from build123d import *

# Parameters (mm, degrees)
ESQUISSE1_W                  = 50
ESQUISSE1_H                  = 100
BOSS_EXTRU_1_DEPTH           = 51.25
ESQUISSE2_W                  = 40
ESQUISSE2_H                  = 40
ESQUISSE2_W_2                = 20
ESQUISSE2_H_2                = 20
BOSS_EXTRU_2_DEPTH           = 45.5
BOSS_EXTRU_2_DEPTH_BACK      = 100
ESQUISSE2_3_W                = 40
ESQUISSE2_3_H                = 82.5
ENL_V_MAT_EXTRU_1_DEPTH      = 101
ENL_V_START                  = -2.5
ENL_V_MAT_EXTRU_3_DEPTH      = 49.75
ENL_V_START_2                = 2.5
ENL_V_MAT_EXTRU_4_DEPTH      = 49.75
ESQUISSE1_6_R                = 5
ENL_V_MAT_EXTRU_5_DEPTH      = 52.25
ENL_V_MAT_EXTRU_5_DEPTH_BACK = 52.25
ENL_V_START_3                = -20
ESQUISSE1_7_W                = 20
ESQUISSE1_7_H                = 85.5
ENL_V_MAT_EXTRU_6_DEPTH      = 31.25
ENL_V_START_4                = 20
ESQUISSE1_8_W                = 20
ESQUISSE1_8_H                = 85.5
ENL_V_MAT_EXTRU_7_DEPTH      = 31.25


with BuildPart() as part:
    # Esquisse1 → Boss.-Extru.1 (new body, symmetric)
    with BuildSketch(Plane.XY):
        with Locations((-25, 50)):
            Rectangle(ESQUISSE1_W, ESQUISSE1_H)
    extrude(amount=BOSS_EXTRU_1_DEPTH, both=True)

    # Esquisse2 → Boss.-Extru.2 (add, two sides)
    with BuildSketch(Plane(origin=(0, 100, 0), x_dir=(1, 0, 0), z_dir=(0, 1, 0))) as boss_extru_2_sk:
        Polygon((205, 20), (50, 44.340452261), (50, -44.340452261), (205, -20), (185, -20), (185, 20), align=None)
        Polygon((6, 51.25), (0, 51.25), (0, 41.25), (40, 41.25), (40, -41.25), (0, -41.25), (0, -51.25), (6, -51.25), (50, -44.340452261), (50, 44.340452261), align=None)
        with Locations((205, 0)):
            Rectangle(ESQUISSE2_W, ESQUISSE2_H)
        with Locations((205, 0)):
            Rectangle(ESQUISSE2_W_2, ESQUISSE2_H_2, mode=Mode.SUBTRACT)
    extrude(amount=BOSS_EXTRU_2_DEPTH)
    extrude(boss_extru_2_sk.sketch, amount=-BOSS_EXTRU_2_DEPTH_BACK)

    # Esquisse2_3 → Enl_v. mat.-Extru.1 (cut, through all)
    with BuildSketch(Plane(origin=(0, 100, 0), x_dir=(1, 0, 0), z_dir=(0, 1, 0))):
        with Locations((-20, 0)):
            Rectangle(ESQUISSE2_3_W, ESQUISSE2_3_H)
        with Locations((20, 0)):
            Rectangle(ESQUISSE2_3_W, ESQUISSE2_3_H)
    extrude(amount=-ENL_V_MAT_EXTRU_1_DEPTH, mode=Mode.SUBTRACT)

    # Esquisse1_4 → Enl_v. mat.-Extru.3 (cut, through all)
    with BuildSketch(Plane.XY.offset(ENL_V_START)):
        with BuildLine():
            Line((50, 100), (50, 20))
            Line((50, 20), (65, 20))
            ThreePointArc((65, 20), (72.071067812, 17.071067812), (75, 10))
            Line((75, 10), (75, 6))
            Line((75, 6), (103.975092222, 6))
            ThreePointArc((103.975092222, 6), (108.20127484, 6.93692213), (111.635536654, 9.572123903))
            Line((111.635536654, 9.572123903), (139.204786201, 42.427876097))
            ThreePointArc((139.204786201, 42.427876097), (142.639048015, 45.06307787), (146.865230633, 46))
            Line((146.865230633, 46), (165, 46))
            Line((165, 46), (165, 50))
            ThreePointArc((165, 50), (167.928932188, 57.071067812), (175, 60))
            Line((175, 60), (185, 60))
            Line((185, 60), (185, 145.5))
            Line((185, 145.5), (171.285964092, 145.5))
            ThreePointArc((171.285964092, 145.5), (167.059781475, 144.56307787), (163.625519661, 141.927876097))
            Line((163.625519661, 141.927876097), (131.441222142, 103.572123903))
            ThreePointArc((131.441222142, 103.572123903), (128.006960328, 100.93692213), (123.780777711, 100))
            Line((123.780777711, 100), (50, 100))
        make_face()
    extrude(amount=-ENL_V_MAT_EXTRU_3_DEPTH, mode=Mode.SUBTRACT)

    # Esquisse1_5 → Enl_v. mat.-Extru.4 (cut, through all)
    with BuildSketch(Plane.XY.offset(ENL_V_START_2)):
        with BuildLine():
            Line((50, 100), (50, 20))
            Line((50, 20), (65, 20))
            ThreePointArc((65, 20), (72.071067812, 17.071067812), (75, 10))
            Line((75, 10), (75, 6))
            Line((75, 6), (103.975092222, 6))
            ThreePointArc((103.975092222, 6), (108.20127484, 6.93692213), (111.635536654, 9.572123903))
            Line((111.635536654, 9.572123903), (139.204786201, 42.427876097))
            ThreePointArc((139.204786201, 42.427876097), (142.639048015, 45.06307787), (146.865230633, 46))
            Line((146.865230633, 46), (165, 46))
            Line((165, 46), (165, 50))
            ThreePointArc((165, 50), (167.928932188, 57.071067812), (175, 60))
            Line((175, 60), (185, 60))
            Line((185, 60), (185, 145.5))
            Line((185, 145.5), (171.285964092, 145.5))
            ThreePointArc((171.285964092, 145.5), (167.059781475, 144.56307787), (163.625519661, 141.927876097))
            Line((163.625519661, 141.927876097), (131.441222142, 103.572123903))
            ThreePointArc((131.441222142, 103.572123903), (128.006960328, 100.93692213), (123.780777711, 100))
            Line((123.780777711, 100), (50, 100))
        make_face()
    extrude(amount=ENL_V_MAT_EXTRU_4_DEPTH, mode=Mode.SUBTRACT)

    # Esquisse1_6 → Enl_v. mat.-Extru.5 (cut, two sides)
    with BuildSketch(Plane.XY) as enl_v_mat_extru_5_sk:
        with BuildLine():
            Line((0, 100), (50, 100))
            Line((50, 100), (123.780777711, 100))
            ThreePointArc((123.780777711, 100), (128.006960328, 100.93692213), (131.441222142, 103.572123903))
            Line((131.441222142, 103.572123903), (163.625519661, 141.927876097))
            ThreePointArc((163.625519661, 141.927876097), (167.059781475, 144.56307787), (171.285964092, 145.5))
            Line((171.285964092, 145.5), (0, 145.5))
            Line((0, 145.5), (0, 100))
        make_face()
        with BuildLine():
            ThreePointArc((114.433382603, 3.572123903), (110.999120789, 0.93692213), (106.772938171, 0))
            Line((106.772938171, 0), (225, 0))
            Line((225, 0), (225, 40))
            Line((225, 40), (205, 40))
            Line((205, 40), (149.663076582, 40))
            ThreePointArc((149.663076582, 40), (145.436893964, 39.06307787), (142.00263215, 36.427876097))
            Line((142.00263215, 36.427876097), (114.433382603, 3.572123903))
        make_face()
        with Locations((65, 10)):
            Circle(ESQUISSE1_6_R)
        with Locations((175, 50)):
            Circle(ESQUISSE1_6_R)
    extrude(amount=ENL_V_MAT_EXTRU_5_DEPTH, mode=Mode.SUBTRACT)
    extrude(enl_v_mat_extru_5_sk.sketch, amount=-ENL_V_MAT_EXTRU_5_DEPTH_BACK, mode=Mode.SUBTRACT)

    # Esquisse1_7 → Enl_v. mat.-Extru.6 (cut)
    with BuildSketch(Plane.XY.offset(ENL_V_START_3)):
        with Locations((195, 102.75)):
            Rectangle(ESQUISSE1_7_W, ESQUISSE1_7_H)
    extrude(amount=-ENL_V_MAT_EXTRU_6_DEPTH, mode=Mode.SUBTRACT)

    # Esquisse1_8 → Enl_v. mat.-Extru.7 (cut)
    with BuildSketch(Plane.XY.offset(ENL_V_START_4)):
        with Locations((195, 102.75)):
            Rectangle(ESQUISSE1_8_W, ESQUISSE1_8_H)
    extrude(amount=ENL_V_MAT_EXTRU_7_DEPTH, mode=Mode.SUBTRACT)


solid = part.part
Can you work these out from the model? Positions are in its coordinate system, mm. A direction names the side the tool comes from. Coordinates: 2 decimals unless noted, no trailing zeros. Order: outer loops, then holes, each group sorted by start corner. A loop starts at its lowest first (then second) coordinate and runs counter-clockwise, first axis right, second up. Notation, with made-up numbers: (18, -24.75) - (66, -24.75) arc R18 cw to (66, -16.75) - close; hole circle Ø6 at (26, 29). An arc over 180 degrees is marked (long way). Answer as a JSON object with one key per item and string values. Group by question number.
Q1. Imagine slicing it at C-C (y = 110.5). Please give me the cut outline in (x, z), and give its area (3 significant figures).
Q2. We'd pull the mould along Z, two halves only. Please class faces 1 (the face through (215, 93, 0)), 2 (the face through (89, 6, -21)): +Z half, -Z half, draft (parallel to the pull), parting line (faces both ways), or undercut.
Q3. I need wall thicknesses on line 1 (X direction, y = 96, z = -17.5); line 2 (X direction, y = 96.5, z = -2); line 3 (X direction, y = 50, z = 3). Which ranges of each line are inside material? Lowest first, please. Write a range as from..to.
Q4. Imagine slicing it at D-D (x = 54.5). Please give me the cut outline in (y, z).
Q5. Will these pins go through, and if not, where does the flat tip stop? P1, Ø5, axis at y = 15.5, z = 0.5, coming from the +X side; P2, Ø3, axis at x = 16.5, y = 85, coming from the -Z side; P3, Ø20, axis at x = 153.5, z = 22, coming from the +Y side.
Q6. Imagine slicing it at B-B (y = 69). Please give me the cut outline in (x, z).
Q7. On a 3-axis mill with a long thin cutter (end or side, diameter ignored), from which of +Z, -Z, +X, -X, +Y, -Y can I reach the whole of each face in a straight line? I mean faces 3 (the face through (185, 102, -11)), 4 (the face through (179, 40, 0)), 5 (the face through (108.146, 6.911, 18.949)), 6 (the face through (195, 93, 0)), 7 (the face through (171, 53, 0)). Say none if no direction works.
Q8. Imagine slicing it at A-A (z = -6). Give the number of separate pieces and of enclosed holes in the cut face, and give its area (3 significant figures).
Determined:
{
 "1": {"outline": "(137.25, -2.5) - (185, -2.5) - (185, -20) - (225, -20) - (225, 20) - (185, 20) - (185, 2.5) - (137.25, 2.5) - close; hole (195, -10) - (215, -10) - (215, 10) - (195, 10) - close", "area": "1,440 mm2"},
 "2": {"face 1": "undercut", "face 2": "draft"},
 "3": {"line 1": "x = -50..-40, 40..50, 185..225", "line 2": "x = -50..-40, 40..195, 215..225", "line 3": "x = -50..-40, 40..50, 165..170, 180..195, 215..225"},
 "4": {"outline": "(0, -43.63) - (20, -43.63) - (20, -2.5) - (100, -2.5) - (100, 2.5) - (20, 2.5) - (20, 43.63) - (0, 43.63) - close"},
 "5": {"P1": "stops at x = 126.54", "P2": "stops at z = -49.84", "P3": "stops at y = 46"},
 "6": {"outline": "(-50, -51.25) - (6, -51.25) - (50, -44.34) - (50, -2.5) - (185, -2.5) - (185, -20) - (225, -20) - (225, 20) - (185, 20) - (185, 2.5) - (50, 2.5) - (50, 44.34) - (6, 51.25) - (-50, 51.25) - close; hole (-40, -41.25) - (40, -41.25) - (40, 41.25) - (-40, 41.25) - close; hole (195, -10) - (215, -10) - (215, 10) - (195, 10) - close"},
 "7": {"face 3": "-Z, +Y", "face 4": "+Z, -Z, +X, -Y", "face 5": "+Z, +Y", "face 6": "+Y, -Y", "face 7": "+Z, -Z"},
 "8": {"separate pieces": "3", "enclosed holes": "2", "area": "5,460 mm2"}
}
